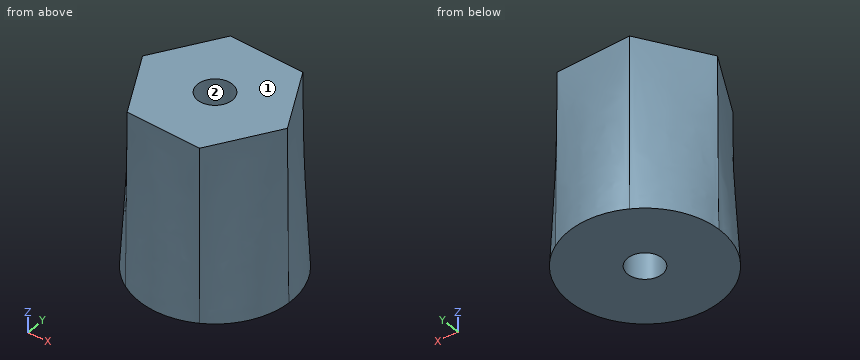
```python
from build123d import *

# Parameters (mm, degrees)
F4_R     = 15
F5_DEPTH = 208


# Not quite as in the source:
# - the arcs of a loft's sections are written as splines that run evenly, so that the points pair up as in the source's solid


with BuildPart() as f3:
    # F2 (on offset) → F3 section 0
    with BuildSketch(Plane.XY.offset(150)):
        Polygon((29.4808263494, -57.1909035932), (64.2691885518, -3.0643072535), (34.7883622024, 54.1265963397), (-29.4808263494, 57.1909035932), (-64.2691885518, 3.0643072535), (-34.7883622024, -54.1265963397), align=None)
    # F1 (on Top) → F3 section 1
    with BuildSketch(Plane.XY):
        with BuildLine():
            add(Edge.make_bspline(
                [(30.0460333415, -58.2873687402), (33.4370549976, -56.5393613769), (36.6750958203, -54.4947096368), (42.7470280691, -49.8741177675), (45.5808257272, -47.2982489935), (50.7581543238, -41.6934743272), (53.1016053094, -38.6646549886), (57.2270197442, -32.2459957674), (59.008919485, -28.8562550072), (61.9570711279, -21.8187389434), (63.123277502, -18.1710723193), (64.8045882572, -10.7285307775), (65.319666674, -6.933770794), (65.5013587195, -3.1230562134)],
                knots=[0, 0, 0, 0, 0.1666666667, 0.1666666667, 0.3333333333, 0.3333333333, 0.5, 0.5, 0.6666666667, 0.6666666667, 0.8333333333, 0.8333333333, 1, 1, 1, 1], degree=3))
            add(Edge.make_bspline(
                [(65.5013587195, -3.1230562134), (65.683050765, 0.6876583672), (65.5313508275, 4.5142098482), (64.5657670125, 12.0829533604), (63.7518980465, 15.8250285085), (61.4866851013, 23.11111393), (60.0353761034, 26.6550116854), (56.5393613769, 33.4370549976), (54.4947096368, 36.6750958203), (49.8741177675, 42.7470280691), (47.2982489935, 45.5808257272), (41.6934743272, 50.7581543238), (38.6646549886, 53.1016053094), (35.455325378, 55.1643125268)],
                knots=[0, 0, 0, 0, 0.1666666667, 0.1666666667, 0.3333333333, 0.3333333333, 0.5, 0.5, 0.6666666667, 0.6666666667, 0.8333333333, 0.8333333333, 1, 1, 1, 1], degree=3))
            add(Edge.make_bspline(
                [(35.455325378, 55.1643125268), (32.2459957674, 57.2270197442), (28.8562550072, 59.008919485), (21.8187389434, 61.9570711279), (18.1710723193, 63.123277502), (10.7285307775, 64.8045882572), (6.933770794, 65.319666674), (-0.6876583672, 65.683050765), (-4.5142098482, 65.5313508275), (-12.0829533604, 64.5657670125), (-15.8250285085, 63.7518980465), (-23.11111393, 61.4866851013), (-26.6550116854, 60.0353761034), (-30.0460333415, 58.2873687402)],
                knots=[0, 0, 0, 0, 0.1666666667, 0.1666666667, 0.3333333333, 0.3333333333, 0.5, 0.5, 0.6666666667, 0.6666666667, 0.8333333333, 0.8333333333, 1, 1, 1, 1], degree=3))
            add(Edge.make_bspline(
                [(-30.0460333415, 58.2873687402), (-33.4370549976, 56.5393613769), (-36.6750958203, 54.4947096368), (-42.7470280691, 49.8741177675), (-45.5808257272, 47.2982489935), (-50.7581543238, 41.6934743272), (-53.1016053094, 38.6646549886), (-57.2270197442, 32.2459957674), (-59.008919485, 28.8562550072), (-61.9570711279, 21.8187389434), (-63.123277502, 18.1710723193), (-64.8045882572, 10.7285307775), (-65.319666674, 6.933770794), (-65.5013587195, 3.1230562134)],
                knots=[0, 0, 0, 0, 0.1666666667, 0.1666666667, 0.3333333333, 0.3333333333, 0.5, 0.5, 0.6666666667, 0.6666666667, 0.8333333333, 0.8333333333, 1, 1, 1, 1], degree=3))
            add(Edge.make_bspline(
                [(-65.5013587195, 3.1230562134), (-65.683050765, -0.6876583672), (-65.5313508275, -4.5142098482), (-64.5657670125, -12.0829533604), (-63.7518980465, -15.8250285085), (-61.4866851013, -23.11111393), (-60.0353761034, -26.6550116854), (-56.5393613769, -33.4370549976), (-54.4947096368, -36.6750958203), (-49.8741177675, -42.7470280691), (-47.2982489935, -45.5808257272), (-41.6934743272, -50.7581543238), (-38.6646549886, -53.1016053094), (-35.455325378, -55.1643125268)],
                knots=[0, 0, 0, 0, 0.1666666667, 0.1666666667, 0.3333333333, 0.3333333333, 0.5, 0.5, 0.6666666667, 0.6666666667, 0.8333333333, 0.8333333333, 1, 1, 1, 1], degree=3))
            add(Edge.make_bspline(
                [(-35.455325378, -55.1643125268), (-32.2459957674, -57.2270197442), (-28.8562550072, -59.008919485), (-21.8187389434, -61.9570711279), (-18.1710723193, -63.123277502), (-10.7285307775, -64.8045882572), (-6.933770794, -65.319666674), (0.6876583672, -65.683050765), (4.5142098482, -65.5313508275), (12.0829533604, -64.5657670125), (15.8250285085, -63.7518980465), (23.11111393, -61.4866851013), (26.6550116854, -60.0353761034), (30.0460333415, -58.2873687402)],
                knots=[0, 0, 0, 0, 0.1666666667, 0.1666666667, 0.3333333333, 0.3333333333, 0.5, 0.5, 0.6666666667, 0.6666666667, 0.8333333333, 0.8333333333, 1, 1, 1, 1], degree=3))
        make_face()
    loft(ruled=True)

    # F4 (on face) → F5 (cut)
    with BuildSketch(Plane(origin=(0, 0, 0), x_dir=(1, 0, 0), z_dir=(0, 0, -1))):
        Circle(F4_R)
    extrude(amount=-F5_DEPTH, mode=Mode.SUBTRACT)


solid = f3.part
```
The model under review builds one solid part; all positions refer to its coordinate system, in mm. Face numbers are marked on the shaded views. Round coordinates to 2 decimals unless told otherwise and drop trailing zeros.
Item 1: For line 1 (X direction, y = 0, z = 46); line 2 (X direction, y = 0, z = 80); line 3 (Y direction, x = 9, z = 38), list the stretches that pass through material, from the lowest coordinate up.
Determined:
line 1: x = -64.74 to -15, 15 to 64.74
line 2: x = -64.1 to -15, 15 to 64.1
line 3: y = -62.73 to -12, 12 to 62.51
Item 2: Clearance check with flat-ended pins moving along their axes: pin 1 Ø12 at (y, z) = (21, 74.5) entering from -X; pin 2 Ø3 at (y, z) = (0, 91) entering from +X; pin 3 Ø1.5 at (x, z) = (22.5, 27) entering from +Y. State where each tip first meets the part, or that it passes through.
Determined:
pin 1: stops at x = -60.53
pin 2: stops at x = 64.32
pin 3: stops at y = 60.53
Item 3: Mouldability with a two-part tool opening along Y and no side actions: class the marked faces 1 and 2 as released by +Y, released by -Y, zero draft, split by the parting line, or undercut.
Determined:
face 1: zero draft
face 2: undercut
